Part model, mm, in its own coordinate system. Coordinates: 2 decimals unless noted, no trailing zeros. Loops run counter-clockwise (first coordinate to the right, second up) from the corner with the lowest first, then second, coordinate; pieces in that order, holes last.
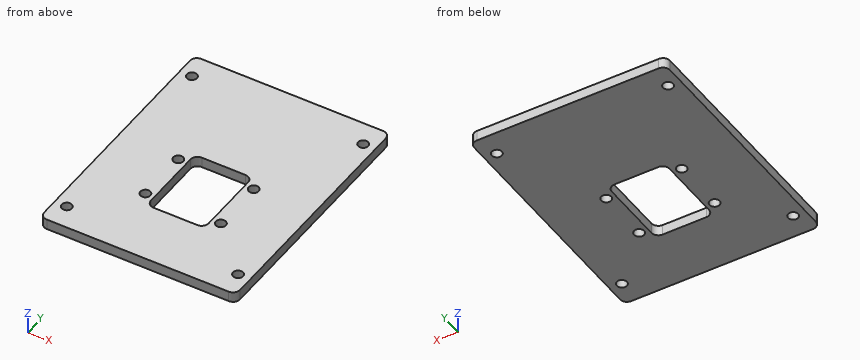
```python
from build123d import *

# Parameters (mm, degrees)
SKETCH1_W           = 56.02
SKETCH1_H           = 71.58
SKETCH1_R           = 1.45
SKETCH1_W_2         = 16.51
SKETCH1_H_2         = 22.32
BOSS_EXTRUDE1_DEPTH = 3
FILLET1_R           = 2


with BuildPart() as part:
    # Sketch1 → Boss-Extrude1 (new body)
    with BuildSketch(Plane.XY):
        with Locations((0, 7.16)):
            Rectangle(SKETCH1_W, SKETCH1_H)
        with Locations((-10.795, -7.62)):
            Circle(SKETCH1_R, mode=Mode.SUBTRACT)
        with Locations((-10.795, 7.62)):
            Circle(SKETCH1_R, mode=Mode.SUBTRACT)
        with Locations((10.795, 7.62)):
            Circle(SKETCH1_R, mode=Mode.SUBTRACT)
        with Locations((10.795, -7.62)):
            Circle(SKETCH1_R, mode=Mode.SUBTRACT)
        with Locations((24.5, -21.84)):
            Circle(SKETCH1_R, mode=Mode.SUBTRACT)
        with Locations((-24.5, 36.16)):
            Circle(SKETCH1_R, mode=Mode.SUBTRACT)
        with Locations((-24.5, -21.84)):
            Circle(SKETCH1_R, mode=Mode.SUBTRACT)
        with Locations((24.5, 36.16)):
            Circle(SKETCH1_R, mode=Mode.SUBTRACT)
        Rectangle(SKETCH1_W_2, SKETCH1_H_2, mode=Mode.SUBTRACT)
    extrude(amount=BOSS_EXTRUDE1_DEPTH)

    # Fillet1
    fillet1_edges = [part.edges().sort_by_distance(p)[0] for p in [
        (-8.255, 11.16, 1.5),
        (-8.255, -11.16, 1.5),
        (8.255, -11.16, 1.5),
        (8.255, 11.16, 1.5),
        (-28.01, 42.95, 1.5),
        (28.01, 42.95, 1.5),
        (28.01, -28.63, 1.5),
        (-28.01, -28.63, 1.5),
    ]]
    fillet(fillet1_edges, radius=FILLET1_R)


solid = part.part
```
Q1. Saw through at C-C (y = -7.62). List the corners of the cut face in (x, z) (3 decimals), plus the area to 3 significant figures.
Q2. Saw through at B-B (z = 1.45). Count the separate pieces of the cut face and the enclosed holes in it, plus the area to 3 significant figures.
Q3. Probe line 1 (Y direction, x = 24.5, z = 1.45); line 2 (X direction, y = -2.5, z = 0.6) (3 decimals); line 3 (X direction, y = -8, z = 1.5) (3 decimals). List the from-to ranges inside material, lowest first.
Q4. Saw through at A-A (y = 36.16). List the corners of the cut face in (x, z), plus the area to 3 significant figures.
Q5. Drop a flat-ended pin along its axis: P1, Ø2.5, axis at x = -10.795, y = 7.62, coming from the +Z side. Give the stop position or say it passes through.
Checked values:
1. outline: (-28.01, 0) - (-12.245, 0) - (-12.245, 3) - (-28.01, 3) - close; (-9.345, 0) - (-8.255, 0) - (-8.255, 3) - (-9.345, 3) - close; (8.255, 0) - (9.345, 0) - (9.345, 3) - (8.255, 3) - close; (12.245, 0) - (28.01, 0) - (28.01, 3) - (12.245, 3) - close
1. area: 101 mm2
2. separate pieces: 1
2. enclosed holes: 9
2. area: 3,590 mm2
3. line 1: y = -28.63 to -23.29, -20.39 to 34.71, 37.61 to 42.95
3. line 2: x = -28.01 to -8.255, 8.255 to 28.01
3. line 3: x = -28.01 to -12.194, -9.396 to -8.255, 8.255 to 9.396, 12.194 to 28.01
4. outline: (-28.01, 0) - (-25.95, 0) - (-25.95, 3) - (-28.01, 3) - close; (-23.05, 0) - (23.05, 0) - (23.05, 3) - (-23.05, 3) - close; (25.95, 0) - (28.01, 0) - (28.01, 3) - (25.95, 3) - close
4. area: 151 mm2
5. P1: passes through
